```python
from build123d import *

# Parameters (mm, degrees)
BOSS_EXTRUDE3_DEPTH   = 14.5
SKETCH8_R             = 7.935
CUT_EXTRUDE3_DEPTH    = 88
CUT_EXTRUDE7_DEPTH    = 2.4
CUT_EXTRUDE8_DEPTH    = 2.4
F_1_0MM_DOWEL_HOLE1_D = 3.5
CUT_EXTRUDE10_DEPTH   = 22.4


with BuildPart() as part:
    # Sketch6 → Boss-Extrude3 (new body)
    with BuildSketch(Plane(origin=(0, 0, 0), x_dir=(1, 0, 0), z_dir=(0, 1, 0))):
        Polygon((-21.836914056, -7.954033585), (8.163085944, -7.954033585), (23.163085944, -49.166194877), (-36.836914056, -49.166194877), align=None)
    extrude(amount=BOSS_EXTRUDE3_DEPTH)

    # Sketch8 → Cut-Extrude3 (cut)
    with BuildSketch(Plane.XY.offset(49.166194877)):
        with Locations((-6.836914056, 0)):
            Circle(SKETCH8_R)
    extrude(amount=-CUT_EXTRUDE3_DEPTH, mode=Mode.SUBTRACT)

    # Sketch16 → Cut-Extrude7 (cut)
    with BuildSketch(Plane(origin=(0, 14.5, 0), x_dir=(1, 0, 0), z_dir=(0, 1, 0))):
        Polygon((-26.489739818, -46.452561466), (-23.539739818, -44.749378171), (-23.539739818, -41.343011583), (-26.489739818, -39.639828289), (-29.439739818, -41.343011583), (-29.439739818, -44.749378171), align=None)
        Polygon((12.815911706, -46.452561466), (15.765911706, -44.749378171), (15.765911706, -41.343011583), (12.815911706, -39.639828289), (9.865911706, -41.343011583), (9.865911706, -44.749378171), align=None)
    extrude(amount=-CUT_EXTRUDE7_DEPTH, mode=Mode.SUBTRACT)

    # Sketch17 → Cut-Extrude8 (cut)
    with BuildSketch(Plane.XZ):
        Polygon((-26.489739818, 39.639828289), (-23.539739818, 41.343011583), (-23.539739818, 44.749378171), (-26.489739818, 46.452561466), (-29.439739818, 44.749378171), (-29.439739818, 41.343011583), align=None)
        Polygon((12.815911706, 39.639828289), (15.765911706, 41.343011583), (15.765911706, 44.749378171), (12.815911706, 46.452561466), (9.865911706, 44.749378171), (9.865911706, 41.343011583), align=None)
    extrude(amount=-CUT_EXTRUDE8_DEPTH, mode=Mode.SUBTRACT)

    # Ø1.0mm Dowel Hole1 (through all)
    with Locations(Plane(origin=(-26.489739818, 14.5, 43.046194877), x_dir=(0, 0, 1), z_dir=(0, 1, 0))):
        with Locations((0, 0), (0, 39.305651524)):
            Hole(F_1_0MM_DOWEL_HOLE1_D / 2)

    # Sketch20 → Cut-Extrude10 (cut)
    with BuildSketch(Plane(origin=(0, 14.5, 0), x_dir=(1, 0, 0), z_dir=(0, 1, 0))):
        Polygon((-32.09934406, -36.149828289), (18.425515948, -36.149828289), (8.163085944, -7.954033585), (-21.836914056, -7.954033585), align=None)
    extrude(amount=-CUT_EXTRUDE10_DEPTH, mode=Mode.SUBTRACT)


solid = part.part
```
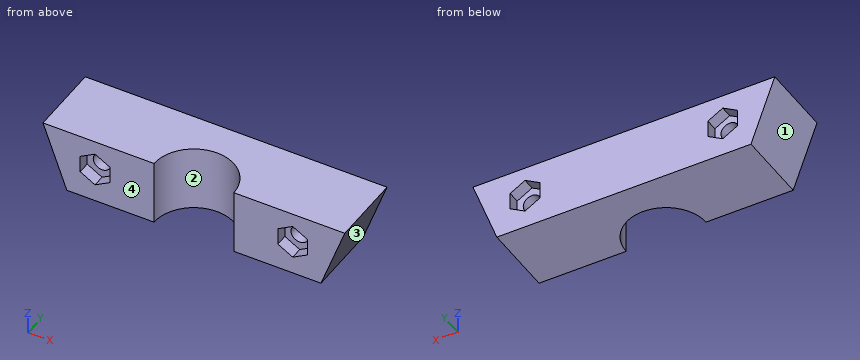
Geometry check sheet. Reference: the model listing, model coordinates, mm. Face numbers are marked on the shaded views. Round coordinates to 2 decimals unless told otherwise and drop trailing zeros. Loops run counter-clockwise (first coordinate to the right, second up) from the corner with the lowest first, then second, coordinate; pieces in that order, holes last. Notation, with made-up numbers: (38, 23.5) -> (47, 23.5) arc R22 cw to (47, 59.5) -> close; hole circle Ø7 at (18, 79.25). An arc over 180 degrees is marked (long way). Use a Markdown table: item, result.
(1) Sectioned sample at D-D (x = -33). Enter the section's corners in (y, z).
Calculated:
| item | result |
|---|---|
| outline | (0, 38.62) -> (14.5, 38.62) -> (14.5, 49.17) -> (0, 49.17) -> close |
(2) Sectioned sample at B-B (z = 42). Give the number of separate pieces and of enclosed holes in the cut face, then the cut area to 3 significant figures.
Calculated:
| item | result |
|---|---|
| separate pieces | 3 |
| enclosed holes | 0 |
| area | 584 mm² |
(3) Scan lines: probe 1 along X at (y, z) = (11, 43); probe 2 along X at (y, z) = (11.5, 42); probe 3 along Y at (x, z) = (-24.5, 42.75). Record each from-to range of solid material in increasing order.
Calculated:
| item | result |
|---|---|
| probe 1 | -34.59 to -28.24, -24.74 to 11.07, 14.57 to 20.92 |
| probe 2 | -34.23 to -27.89, -25.09 to 11.41, 14.22 to 20.55 |
| probe 3 | 2.4 to 12.1 |
(4) Sectioned sample at C-C (y = 11.5). Enter the section's corners in (x, z).
Calculated:
| item | result |
|---|---|
| outline | (-36.84, 49.17) -> (-32.1, 36.15) -> (18.43, 36.15) -> (23.16, 49.17) -> close; hole circle Ø3.5 at (-26.49, 43.05); hole circle Ø3.5 at (12.82, 43.05) |
(5) Go/stop test with flat-tipped pins: P1, Ø4.5, axis at x = 12.5, z = 43, coming from the -Y side; P2, Ø1.9, axis at y = 1, z = 43, coming from the +X side; P3, Ø0.7, axis at y = 14, z = 43.5, coming from the -X side; P4, Ø3, axis at x = -26.49, z = 43.05, coming from the -Y side. Record where each tip stops, or that it passes through.
Calculated:
| item | result |
|---|---|
| P1 | y = 2.4 |
| P2 | x = 21.26 |
| P3 | x = -34.9 |
| P4 | through |
(6) Mould release check, pull along X, two halves, no side actions. Record for the marked faces 1, 2, 3 and 4: released by +X, released by -X, zero draft, split by the parting line, or undercut.
Calculated:
| item | result |
|---|---|
| face 1 | released by -X |
| face 2 | undercut |
| face 3 | released by +X |
| face 4 | zero draft |
(7) Sectioned sample at A-A (y = 3.5). Enter the section's corners in (x, z), then the cut area to 3 significant figures.
Calculated:
| item | result |
|---|---|
| outline | (-36.84, 49.17) -> (-32.1, 36.15) -> (-13.96, 36.15) -> (-13.96, 49.17) -> close; (0.28, 36.15) -> (18.43, 36.15) -> (23.16, 49.17) -> (0.28, 49.17) -> close; hole circle Ø3.5 at (-26.49, 43.05); hole circle Ø3.5 at (12.82, 43.05) |
| area | 515 mm² |
